Verification items for the finished model (mm, model axes). A direction names the side the tool comes from. Round coordinates to 2 decimals unless told otherwise and drop trailing zeros. Write each loop counter-clockwise with the first axis right and the second up, starting at its lowest first coordinate (ties: lowest second). Pieces come first, ordered by that corner, then holes.
from build123d import *

# Parameters (mm, degrees)
BOSS_EXTRUDE1_DEPTH = 180
SKETCH2_R           = 2.6
CUT_EXTRUDE1_DEPTH  = 211
SKETCH2_3_R         = 4.5
CUT_EXTRUDE2_DEPTH  = 6
SKETCH3_R           = 3.05
CUT_EXTRUDE3_DEPTH  = 8
FILLET4_R           = 10
CHAMFER1_SIZE       = 1
FILLET5_R           = 1.5
SKETCH4_W           = 40
SKETCH4_H           = 10
BOSS_EXTRUDE2_DEPTH = 13
CHAMFER2_SIZE       = 13


# Some blends are built 0.0001 mm under size
with BuildPart() as part:
    # Sketch1 → Boss-Extrude1 (new body)
    with BuildSketch(Plane.XY):
        Polygon((0, 10), (0, 0), (90, 0), (90, 45), (19, 45), (19, 70), (16, 70), (16, 64), (4, 64), (4, 35), (75, 35), (75, 10), align=None)
    extrude(amount=BOSS_EXTRUDE1_DEPTH)

    # Sketch2 → Cut-Extrude1 (cut, through all)
    with BuildSketch(Plane(origin=(0, 10, 0), x_dir=(1, 0, 0), z_dir=(0, 1, 0))):
        with Locations(Location((11, -65, 0), (0, 0, 270))):
            Circle(SKETCH2_R)
        with Locations(Location((11, -15, 0), (0, 0, 270))):
            Circle(SKETCH2_R)
        with Locations(Location((11, -115, 0), (0, 0, 270))):
            Circle(SKETCH2_R)
        with Locations(Location((11, -165, 0), (0, 0, 270))):
            Circle(SKETCH2_R)
    extrude(amount=-CUT_EXTRUDE1_DEPTH, mode=Mode.SUBTRACT)

    # Sketch2<3> → Cut-Extrude2 (cut)
    with BuildSketch(Plane(origin=(0, 10, 0), x_dir=(1, 0, 0), z_dir=(0, 1, 0))):
        with Locations(Location((11, -65, 0), (0, 0, 270))):
            Circle(SKETCH2_3_R)
        with Locations(Location((11, -15, 0), (0, 0, 270))):
            Circle(SKETCH2_3_R)
        with Locations(Location((11, -115, 0), (0, 0, 270))):
            Circle(SKETCH2_3_R)
        with Locations(Location((11, -165, 0), (0, 0, 270))):
            Circle(SKETCH2_3_R)
    extrude(amount=-CUT_EXTRUDE2_DEPTH, mode=Mode.SUBTRACT)

    # Sketch3 → Cut-Extrude3 (cut)
    with BuildSketch(Plane(origin=(0, 64, 0), x_dir=(1, 0, 0), z_dir=(0, 1, 0))):
        with Locations(Location((10, -90, 0), (0, 0, 270))):
            Circle(SKETCH3_R)
    extrude(amount=-CUT_EXTRUDE3_DEPTH, mode=Mode.SUBTRACT)

    # Fillet4
    fillet4_edges = [part.edges().sort_by_distance(p)[0] for p in [
        (90, 22.5, 180),
        (0, 5, 0),
        (4, 49.5, 0),
        (90, 22.5, 0),
        (75, 10, 90),
        (75, 35, 90),
        (90, 45, 90),
        (90, 0, 90),
        (4, 49.5, 180),
        (0, 5, 180),
    ]]
    fillet(fillet4_edges, radius=FILLET4_R)

    # Chamfer1
    chamfer1_edges = [part.edges().sort_by_distance(p)[0] for p in [
        (10, 64, 86.95),
        (11, 10, 10.5),
        (11, 10, 60.5),
        (11, 10, 110.5),
        (11, 10, 160.5),
    ]]
    chamfer(chamfer1_edges, length=CHAMFER1_SIZE)

    # Fillet5
    fillet5_edges = [part.edges().sort_by_distance(p)[0] for p in [
        (19, 57.5, 0),
        (16, 67, 0),
        (19, 57.5, 180),
        (16, 67, 180),
    ]]
    fillet(fillet5_edges, radius=FILLET5_R - 0.0001)  # a hair under: the kernel refuses the full size

    # Sketch4 → Boss-Extrude2 (add)
    with BuildSketch(Plane.XZ):
        with Locations((60, 5)):
            Rectangle(SKETCH4_W, SKETCH4_H)
        with Locations((60, 175)):
            Rectangle(SKETCH4_W, SKETCH4_H)
    extrude(amount=BOSS_EXTRUDE2_DEPTH)

    # Chamfer2
    # the kernel refuses this chamfer: 13 mm, written as the material it adds along each edge
    with BuildSketch(Plane(origin=(40, 0, 170), x_dir=(0, 0.027495876610586372, -0.9996219169112968), z_dir=(1, 0, 0))) as chamfer2_piece_1_section:
        Polygon((CHAMFER2_SIZE * 0.999621916911, -CHAMFER2_SIZE * 0.0274958766106), (-CHAMFER2_SIZE * 0.0274958766106, -CHAMFER2_SIZE * 0.999621916911), (0, 0), align=None)
    chamfer2_piece_1 = extrude(amount=40, mode=Mode.PRIVATE)
    chamfer2_piece_1 = split(chamfer2_piece_1, bisect_by=Plane(origin=(60, -13, 165.704745994), z_dir=(0, 1, 0)), keep=Keep.TOP, mode=Mode.PRIVATE)
    add(chamfer2_piece_1)


solid = part.part
Q1. Sectioned sample at B-B (x = 25). Enter the section's corners in (y, z), plus the area to 3 significant figures.
Recorded:
outline: (0, 0) - (10, 0) - (10, 180) - (0, 180) - close; (35, 0) - (45, 0) - (45, 180) - (35, 180) - close
area: 3,600 mm2
Q2. Sectioned sample at A-A (z = 65). Enter the section's corners in (x, y).
Recorded:
outline: (0, 0) - (8.4, 0) - (8.4, 4) - (6.5, 4) - (6.5, 9) - (5.5, 10) - (0, 10) - close; (4, 35) - (65, 35) arc R10 cw to (75, 25) - (75, 20) arc R10 cw to (65, 10) - (16.5, 10) - (15.5, 9) - (15.5, 4) - (13.6, 4) - (13.6, 0) - (80, 0) arc R10 ccw to (90, 10) - (90, 35) arc R10 ccw to (80, 45) - (19, 45) - (19, 70) - (16, 70) - (16, 64) - (4, 64) - close
Q3. Material ranges on line 1 along Y through (x, z) = (15, 68); line 2 along Y through (x, z) = (30.5, 90); line 3 along X through (y, z) = (-1, 8.5), recorded low to high.
Recorded:
line 1: y = 0 to 9.5, 35 to 64
line 2: y = 0 to 10, 35 to 45
line 3: x = 40 to 80
Q4. Release check for a two-part mould opening along X. For faces 1 (the flat face through (9, 4, 17)), 2 (the flat face through (80, -5, 171)), 3 (the flat face through (40, -6, 5)), 4 (the flat face through (39, 0, 89)) record: released by +X, released by -X, zero draft, split by the parting line, or undercut.
Recorded:
face 1: undercut
face 2: released by +X
face 3: released by -X
face 4: zero draft
Q5. Depth check by flat-ended pin: P1, Ø8, axis at y = 34.5, z = 116, coming from the -X side; P2, Ø8, axis at y = 60, z = 56, coming from the +X side; P3, Ø8, axis at y = -7.5, z = 3.5, coming from the +X side. Enter the tip coordinate at first touch or a pass-through.
Recorded:
P1: stops at x = 4
P2: stops at x = 19
P3: stops at x = 80
Q6. Sectioned sample at D-D (z = 90). Enter the section's corners in (x, y).
Recorded:
outline: (0, 0) - (80, 0) arc R10 ccw to (90, 10) - (90, 35) arc R10 ccw to (80, 45) - (19, 45) - (19, 70) - (16, 70) - (16, 64) - (14.05, 64) - (13.05, 63) - (13.05, 56) - (6.95, 56) - (6.95, 63) - (5.95, 64) - (4, 64) - (4, 35) - (65, 35) arc R10 cw to (75, 25) - (75, 20) arc R10 cw to (65, 10) - (0, 10) - close
Q7. Sectioned sample at C-C (y = 60). Enter the section's corners in (x, z).
Recorded:
outline: (4, 10) arc R10 ccw to (14, 0) - (17.5, 0) arc R1.5 ccw to (19, 1.5) - (19, 178.5) arc R1.5 ccw to (17.5, 180) - (14, 180) arc R10 ccw to (4, 170) - close; hole circle Ø6.1 at (10, 90)
Q8. Tool access check on faces 5 (the flat face through (60, -6, 10)), 6 (the cylindrical face through (10.134, 59.549, 86.953)), 7 (the cylindrical face through (10, 2, 17.4)), 8 (the flat face through (19, 57, 89)). Record the directions out of +Z, -Z, +X, -X, +Y, -Y that give a thin tool (end or side, any length) a straight path to the whole face; none if there is none.
Recorded:
face 5: +X, -X, -Y
face 6: +Y
face 7: -Y
face 8: +Z, -Z, +X, +Y
